```python
from build123d import *

# Parameters (mm, degrees)
SKETCH1_W           = 101.6
SKETCH1_H           = 210
SKETCH1_R           = 2.1
SKETCH1_R_2         = 10
SKETCH1_R_3         = 4.1
SKETCH1_R_4         = 14.275
BOSS_EXTRUDE1_DEPTH = 6.35


with BuildPart() as part:
    # Sketch1 → Boss-Extrude1 (new body)
    with BuildSketch(Plane(origin=(0, 0, 0), x_dir=(0, 0, -1), z_dir=(1, 0, 0))):
        Rectangle(SKETCH1_W, SKETCH1_H)
        with Locations((-40.513, -98.65)):
            Circle(SKETCH1_R, mode=Mode.SUBTRACT)
        with Locations((40.513, -98.65)):
            Circle(SKETCH1_R, mode=Mode.SUBTRACT)
        with Locations((19.05, -30.15)):
            Circle(SKETCH1_R_2, mode=Mode.SUBTRACT)
        with Locations((37.010512242, -12.189487758)):
            Circle(SKETCH1_R, mode=Mode.SUBTRACT)
        with Locations((1.089487758, -48.110512242)):
            Circle(SKETCH1_R, mode=Mode.SUBTRACT)
        with Locations((1.089487758, -12.189487758)):
            Circle(SKETCH1_R, mode=Mode.SUBTRACT)
        with Locations((37.010512242, -48.110512242)):
            Circle(SKETCH1_R, mode=Mode.SUBTRACT)
        with Locations((-35.8, -21.9)):
            Circle(SKETCH1_R_3, mode=Mode.SUBTRACT)
        with Locations((0, 80)):
            Circle(SKETCH1_R_4, mode=Mode.SUBTRACT)
        with Locations((-40.513, -73.25)):
            Circle(SKETCH1_R, mode=Mode.SUBTRACT)
        with Locations((40.513, -73.25)):
            Circle(SKETCH1_R, mode=Mode.SUBTRACT)
    extrude(amount=BOSS_EXTRUDE1_DEPTH)


solid = part.part
```
Verification items for the finished model (mm, model axes). Round coordinates to 2 decimals unless told otherwise and drop trailing zeros. Write each loop counter-clockwise with the first axis right and the second up, starting at its lowest first coordinate (ties: lowest second). Pieces come first, ordered by that corner, then holes. Notation, with made-up numbers: (37.5, 50.5) -> (53.5, 50.5) arc R16 cw to (53.5, 68.5) -> close; hole circle Ø8 at (47, -6.75). An arc over 180 degrees is marked (long way). Write each question's results on one line, items separated by ' | '. Start each with the question number.
1. Cross-section at C-C (z = 35.8). Enter the section's corners in (x, y), then the cut area to 3 significant figures.
2. Depth check by flat-ended pin: P1, Ø2.5, axis at y = -12.19, z = -37.01, coming from the +X side. Enter the tip coordinate at first touch or a pass-through.
3. Draft check along Y on faces 1 (the cylindrical face through (3.13, -75.3, -40.06)), 2 (the flat face through (3, -1, 50.8)), 3 (the flat face through (3, 105, 1)). Enter one of: +Y half, -Y half, draft (parallel to the pull), parting line (faces both ways), or undercut.
4. Material ranges on probe 1 along Y at (x, z) = (2.25, 35.8); probe 2 along Y at (x, z) = (3, 39); probe 3 along Y at (x, z) = (4.25, 0) (3 decimals), recorded low to high. Write a range as from..to.
5. Cross-section at A-A (z = -19.05). Enter the section's corners in (x, y).
6. Cross-section at B-B (x = 3.5). Count the separate pieces of the cut face and the enclosed holes in it, then the cut area to 3 significant figures.
Solutions:
1) outline: (0, -105) -> (6.35, -105) -> (6.35, -26) -> (0, -26) -> close; (0, -17.8) -> (6.35, -17.8) -> (6.35, 105) -> (0, 105) -> close | area: 1,280 mm2
2) P1: passes through
3) face 1: undercut | face 2: draft | face 3: +Y half
4) probe 1: y = -105..-26, -17.8..105 | probe 2: y = -105..-100.11, -97.19..-74.71, -71.79..-24.46, -19.34..105 | probe 3: y = -105..-49.906, -46.315..-13.985, -10.394..65.725, 94.275..105
5) outline: (0, -105) -> (6.35, -105) -> (6.35, -40.15) -> (0, -40.15) -> close; (0, -20.15) -> (6.35, -20.15) -> (6.35, 105) -> (0, 105) -> close
6) separate pieces: 1 | enclosed holes: 11 | area: 20,200 mm2
